```python
from build123d import *

# Parameters (mm, degrees)
PAD_DEPTH    = 0.375
SKETCH002_R  = 1.5
PAD001_DEPTH = 0.5
SKETCH003_W  = 10
SKETCH003_H  = 0.5
PAD002_DEPTH = 0.375
SKETCH004_R  = 0.75
PAD003_DEPTH = 0.25


with BuildPart() as part:
    # Sketch → Pad (new body, symmetric)
    with BuildSketch(Plane.XY):
        with BuildLine():
            Line((-0.25, 0), (0, 0))
            Line((0, 0), (0.25, 0))
            ThreePointArc((0.25, 0), (8.71609, -20.785997), (29.295895, -29.741667))
            ThreePointArc((29.290002, -30.241667), (30.749948, -30.008839), (29.295895, -29.741667))
            ThreePointArc((-0.25, 0), (8.360454, -21.137467), (29.290002, -30.241667))
        make_face()
    extrude(amount=PAD_DEPTH, both=True)

    # Sketch002 → Pad001 (join)
    with BuildSketch(Plane.XZ):
        Circle(SKETCH002_R)
    extrude(amount=PAD001_DEPTH)

    # Sketch003 → Pad002 (join, symmetric)
    with BuildSketch(Plane.XY):
        with Locations((25, -30)):
            Rectangle(SKETCH003_W, SKETCH003_H)
    extrude(amount=PAD002_DEPTH, both=True)

    # Sphere → Sphere (revolve, cut)
    with BuildSketch(Plane(origin=(30, -30, 0.6925), x_dir=(1, 0, 0), z_dir=(0, -1, 0))):
        with BuildLine():
            ThreePointArc((0, -0.635), (0.635, 0), (0, 0.635))
            Line((0, 0.635), (0, -0.635))
        make_face()
    revolve(axis=Axis((30, -30, 0.6925), (0, 0, 1)), mode=Mode.SUBTRACT)

    # Sketch004 (on DatumPlane) → Pad003 (join, symmetric)
    with BuildSketch(Plane(origin=(20, -30, 0), x_dir=(1, 0, 0), z_dir=(0, -1, 0))):
        Circle(SKETCH004_R)
    extrude(amount=PAD003_DEPTH, both=True)

    # Sphere001 → Sphere001 (revolve, cut)
    with BuildSketch(Plane(origin=(20, -30.5675, 0), x_dir=(1, 0, 0), z_dir=(0, -1, 0))):
        with BuildLine():
            ThreePointArc((0, -0.635), (0.635, 0), (0, 0.635))
            Line((0, 0.635), (0, -0.635))
        make_face()
    revolve(axis=Axis((20, -30.5675, 0), (0, 0, 1)), mode=Mode.SUBTRACT)


solid = part.part
```
The listing builds one solid part. Answer for the finished solid, in the listing's coordinates (mm). A direction names the side the tool comes from. Give positions to 0.01 mm unless a question says otherwise; leave off trailing zeros. Order: outer loops, then holes, each group sorted by start corner. A loop starts at its lowest first (then second) coordinate and runs counter-clockwise, first axis right, second up. Notation, with made-up numbers: M 7.25,-29.5 L 53.25,-29.5 A28 ccw 53.25,2.5 Z; hole C 41.5,-27 d2. An arc over 180 degrees is marked long. Put each result on its own line as item: value. Start each with the question number.
Item 1: Which of the six approach directions +Z, -Z, +X, -X, +Y, -Y give full straight-line access (tool end or side, diameter ignored) to faces 1 (the face through (24, -30.25, 0)), 2 (the face through (0, 0, 0))?
Item 2: Find the intervals of material crossed by line 1 along Y through (x, z) = (17, 0.2); line 2 along Y through (x, z) = (5, -0.3); line 3 along X through (y, z) = (-26.5, -0.3), in increasing order.
Item 3: Flat-ended cylindrical pins translate along their axes: P1, Ø1.6, axis at x = 21.5, z = 0.5, coming from the +Y side; P2, Ø4, axis at x = 16.5, y = -24, coming from the -Z side; P3, Ø4, axis at x = 13.5, y = -25.5, coming from the +Z side (3 decimals); P4, Ø1.6, axis at x = 26, z = 0, coming from the -Y side. Find the tip coordinate at first contact, or state that the pin passes through.
Item 4: The part is cut by section C-C, the plane y = -28. Determine the outline of the cut face in (x, z) (3 decimals), and give its area (3 significant figures).
Item 5: The part is cut by section D-D, the plane y = -5.5. Determine the outline of the cut face in (x, z) (3 decimals).
Answer key:
1. face 1: +Z, -Z, -X, -Y
1. face 2: +Z, -Z, +X, -X, +Y
2. line 1: y = -27.31 to -26.76
2. line 2: y = -17.03 to -16.13
2. line 3: x = 15.41 to 16.48
3. P1: stops at y = -28.26
3. P2: passes through
3. P3: stops at z = 0.375
3. P4: stops at y = -30.25
4. outline: M 18.552,-0.375 L 19.947,-0.375 L 19.947,0.375 L 18.552,0.375 Z
4. area: 1.05 mm²
5. outline: M 0.254,-0.375 L 0.763,-0.375 L 0.763,0.375 L 0.254,0.375 Z
